Check sheet for the modelled part. Datum: model origin and axes. Units: mm. A direction names the side the tool comes from. Round coordinates to 2 decimals unless told otherwise and drop trailing zeros. Order: outer loops, then holes, each group sorted by start corner. A loop starts at its lowest first (then second) coordinate and runs counter-clockwise, first axis right, second up.
Q1. Cross-section at B-B on x = 0. Record the cut outline in (y, z), then the cut area to 3 significant figures.
Q2. Set-up check for faces 1 (the flat face through (20, 80, 0)), 2 (the flat face through (-20, 80, 0)), 3 (the cylindrical face through (14.619, 100.28, 19.236)), 4 (the flat face through (10, 80, -17)): record each of +Z, -Z, +X, -X, +Y, -Y from which the full face is reachable in a straight line by a thin tool's end or side.
Q3. Cross-section at C-C on y = 68. Record the cut outline in (x, z).
Q4. Mould release check, pull along Y, two halves, no side actions. Record for faces 5 (the flat face through (-10, 80, 17)), 6 (the flat face through (10, 80, 17)), 7 (the conical face through (21.147, 144.79, 6.66)), 8 (the cylindrical face through (4.88, 22.18, -37.18)): +Y half, -Y half, draft (parallel to the pull), parting line (faces both ways), or undercut.
Q5. Scan lines: probe 1 along Y at (x, z) = (0, -17); probe 2 along Y at (x, z) = (9.5, -16.5); probe 3 along Z at (x, y) = (6.5, 90). Record each from-to range of solid material in increasing order.
Q6. Cross-section at A-A on y = 113. Record the cut outline in (x, z).
Q7. Depth check by flat-ended pin: P1, Ø1.5, axis at y = 47, z = 30, coming from the -X side; P2, Ø3, axis at x = -19, z = 0.5, coming from the -Y side; P3, Ø12, axis at x = 29.5, z = 16, coming from the +Y side; P4, Ø3, axis at x = 8.5, y = 41.5, coming from the -Z side. Enter the tip coordinate at first touch or a pass-through.
Q8. Cross-section at D-D on y = 11. Record the cut outline in (x, z).
Autodesk Inventor part; units mm, degrees
ref_plane "YZ Plane" through (0, 0, 0) normal (1, 0, 0) x (0, 1, 0)
ref_plane "XZ Plane" through (0, 0, 0) normal (0, 1, 0) x (-1, 0, 0)
ref_plane "XY Plane" through (0, 0, 0) normal (0, 0, 1) x (1, 0, 0)
sketch "Sketch1" plane through (0, 0, 0) normal (0, 1, 0) x (-1, 0, 0)
  circle A0 centre (0, 0) radius 37.5
  dimension "d0" = 75
extrude "Extrusion1" add sketch "Sketch1" along normal blind 50
fillet "Fillet1" radius 5 1 edges at (37.5, 50, 0)
sketch "Sketch2" plane through (0, 50, 0) normal (0, 1, 0) x (1, 0, 0)
  circle A0 centre (0, 0) radius 5
  dimension "d4" = 10
extrude "Extrusion2" add sketch "Sketch2" along normal blind 70
sketch "Sketch3" plane through (0, 120, 0) normal (0, 1, 0) x (1, 0, 0)
  circle A0 centre (0, 0) radius 32.5
  dimension "d7" = 65
ref_plane "Work Plane1" through (0, 150, 0) normal (0, 1, 0) x (1, 0, 0)
sketch "Sketch4" plane through (0, 150, 0) normal (0, 1, 0) x (1, 0, 0)
  circle A0 centre (0, 0) radius 20
  dimension "d9" = 40
loft "Loft1" add profiles "Sketch3", "Sketch4"
sketch "Sketch5" plane through (0, 120, 0) normal (0, -1, 0) x (1, 0, 0)
  circle A0 centre (0, 0) radius 20
  circle A1 centre (-20, 0) radius 5
  circle A2 centre (0, 0) radius 5
  circle A3 centre (-10, -17.3205) radius 5
  circle A4 centre (10, -17.3205) radius 5
  circle A5 centre (20, 0) radius 5
  circle A6 centre (10, 17.3205) radius 5
  circle A7 centre (-10, 17.3205) radius 5
  dimension "d14" = 10
  dimension "d15" = 20
  dimension "d18" = 360
extrude "Extrusion3" add sketch "Sketch5" along normal blind 40 contours A0 A5 | A0 A5 | A6 A0 | A0 A6 | A4 A0 | A0 A4 | A7 A0 | A0 A7 | A3 A0 | A0 A3 | A1 A0 | A0 A1
properties part number "Main_Tower"
Results found:
1. outline: (0, -37.5) - (45, -37.5) arc R5 ccw to (50, -32.5) - (50, -5) - (120, -5) - (120, -32.5) - (150, -20) - (150, 20) - (120, 32.5) - (120, 5) - (50, 5) - (50, 32.5) arc R5 ccw to (45, 37.5) - (0, 37.5) - close
1. area: 6,010 mm2
2. face 1: +Z, -Z, +X
2. face 2: +Z, -Z, -X
2. face 3: none
2. face 4: +Z, -Z, +X, -X
3. outline: circle Ø10 at (0, 0)
4. face 5: undercut
4. face 6: undercut
4. face 7: +Y half
4. face 8: draft
5. probe 1: y = 0 to 50, 120 to 150
5. probe 2: y = 0 to 50, 80 to 150
5. probe 3: z = -20.89 to -13.75, 13.75 to 20.89
6. outline: circle Ø10 at (-20, 0); circle Ø10 at (-10, -17.32); circle Ø10 at (-10, 17.32); circle Ø10 at (0, 0); circle Ø10 at (10, -17.32); circle Ø10 at (10, 17.32); circle Ø10 at (20, 0)
7. P1: stops at x = -22.91
7. P2: stops at y = 0
7. P3: stops at y = 131.86
7. P4: stops at z = -36.84
8. outline: circle Ø75 at (0, 0)
